Can you work these out from the model? Positions are in its coordinate system, mm. A direction names the side the tool comes from. Round coordinates to 2 decimals unless told otherwise and drop trailing zeros. Order: outer loops, then holes, each group sorted by start corner. A loop starts at its lowest first (then second) coordinate and runs counter-clockwise, first axis right, second up. Notation, with made-up numbers: M -16.75,42.5 L 29.25,42.5 A22 ccw 29.25,64.5 Z; hole C -17.75,4 d7. An arc over 180 degrees is marked long. One line per question, with ' | ' between items.
```python
from build123d import *

# Parameters (mm, degrees)
SKIZZE1_R                        = 2.5
AUFSATZ_LINEAR_AUSTRAGEN4_DEPTH  = 1
SKIZZE1_3_R                      = 2.5
SKIZZE1_3_R_2                    = 1.5
AUFSATZ_LINEAR_AUSTRAGEN5_DEPTH  = 10
SKIZZE1_4_R                      = 1.5
AUFSATZ_LINEAR_AUSTRAGEN6_DEPTH  = 12
VERRUNDUNG4_R                    = 1
SKIZZE1_5_W                      = 2
SKIZZE1_5_H                      = 16
AUFSATZ_LINEAR_AUSTRAGEN7_DEPTH  = 12
FASE3_SIZE                       = 12
VERRUNDUNG5_R                    = 12
SCHNITT_LINEAR_AUSTRAGEN2_DEPTH  = 12
SKIZZE5_4_R                      = 4.25
SKIZZE5_4_R_2                    = 3.45
AUFSATZ_LINEAR_AUSTRAGEN10_DEPTH = 6


with BuildPart() as part:
    # Skizze1 → Aufsatz-Linear austragen4 (new body)
    with BuildSketch(Plane.XY):
        with BuildLine():
            Line((-11, 12), (-16.5, 12))
            Line((-16.5, 12), (-16.5, 8))
            ThreePointArc((-16.5, 8), (-14.5, 6), (-16.5, 4))
            Line((-16.5, 4), (-16.5, -30))
            Line((-16.5, -30), (16.5, -30))
            Line((16.5, -30), (16.5, 4))
            ThreePointArc((16.5, 4), (14.5, 6), (16.5, 8))
            Line((16.5, 8), (16.5, 12))
            Line((16.5, 12), (11, 12))
            Line((11, 12), (9, 12))
            Line((9, 12), (9, 28))
            Line((9, 28), (-9, 28))
            Line((-9, 28), (-9, 12))
            Line((-9, 12), (-11, 12))
        make_face()
        with Locations((-11.5, -14)):
            Circle(SKIZZE1_R, mode=Mode.SUBTRACT)
        with Locations((11.5, -14)):
            Circle(SKIZZE1_R, mode=Mode.SUBTRACT)
        with Locations((-11.5, 9)):
            Circle(SKIZZE1_R, mode=Mode.SUBTRACT)
        with Locations((11.5, 9)):
            Circle(SKIZZE1_R, mode=Mode.SUBTRACT)
    extrude(amount=AUFSATZ_LINEAR_AUSTRAGEN4_DEPTH)

    # Skizze1<3> → Aufsatz-Linear austragen5 (add)
    # profile 1 of 4: a face of its own
    with BuildSketch(Plane.XY):
        with Locations((11.5, 9)):
            Circle(SKIZZE1_3_R)
        with Locations((11.5, 9)):
            Circle(SKIZZE1_3_R_2, mode=Mode.SUBTRACT)
    # profile 2 of 4: a face of its own
    with BuildSketch(Plane.XY):
        with Locations((-11.5, 9)):
            Circle(SKIZZE1_3_R)
        with Locations((-11.5, 9)):
            Circle(SKIZZE1_3_R_2, mode=Mode.SUBTRACT)
    # profile 3 of 4: a face of its own
    with BuildSketch(Plane.XY):
        with Locations((-11.5, -14)):
            Circle(SKIZZE1_3_R)
        with Locations((-11.5, -14)):
            Circle(SKIZZE1_3_R_2, mode=Mode.SUBTRACT)
    # profile 4 of 4: a face of its own
    with BuildSketch(Plane.XY):
        with Locations((11.5, -14)):
            Circle(SKIZZE1_3_R)
        with Locations((11.5, -14)):
            Circle(SKIZZE1_3_R_2, mode=Mode.SUBTRACT)
    extrude(amount=AUFSATZ_LINEAR_AUSTRAGEN5_DEPTH)

    # Skizze1<4> → Aufsatz-Linear austragen6 (add)
    with BuildSketch(Plane.XY):
        with Locations((-11.5, 9)):
            Circle(SKIZZE1_4_R)
        with Locations((11.5, 9)):
            Circle(SKIZZE1_4_R)
        with Locations((-11.5, -14)):
            Circle(SKIZZE1_4_R)
        with Locations((11.5, -14)):
            Circle(SKIZZE1_4_R)
    extrude(amount=AUFSATZ_LINEAR_AUSTRAGEN6_DEPTH)

    # Verrundung4
    verrundung4_edges = [part.edges().sort_by_distance(p)[0] for p in [
        (-13, 9, 12),
        (10, 9, 12),
        (-13, -14, 12),
        (10, -14, 12),
    ]]
    fillet(verrundung4_edges, radius=VERRUNDUNG4_R)

    # Skizze1<5> → Aufsatz-Linear austragen7 (add)
    with BuildSketch(Plane.XY):
        with Locations((-10, 20)):
            Rectangle(SKIZZE1_5_W, SKIZZE1_5_H)
        Polygon((11, 30), (-11, 30), (-11, 28), (-9, 28), (9, 28), (11, 28), align=None)
        with Locations((10, 20)):
            Rectangle(SKIZZE1_5_W, SKIZZE1_5_H)
    extrude(amount=AUFSATZ_LINEAR_AUSTRAGEN7_DEPTH)

    # Fase3
    # the kernel refuses this chamfer: 12 mm, written as the material it takes off along each edge
    with BuildSketch(Plane(origin=(-41.860195856, 12, 12), x_dir=(0, -0.027495876610586348, -0.9996219169112968), z_dir=(1, 0, 0))) as fase3_piece_1_section:
        Polygon((FASE3_SIZE * 0.999621916911, FASE3_SIZE * 0.0274958766106), (-FASE3_SIZE * 0.0274958766106, FASE3_SIZE * 0.999621916911), (0, 0), align=None)
    fase3_piece_1 = extrude(amount=63.720391711, mode=Mode.PRIVATE)
    fase3_piece_1 = split(fase3_piece_1, bisect_by=Plane(origin=(-10, 16.015873454, 1), z_dir=(0, 0, 1)), keep=Keep.TOP, mode=Mode.PRIVATE)
    add(fase3_piece_1, mode=Mode.SUBTRACT)
    with BuildSketch(Plane(origin=(-21.860195856, 12, 12), x_dir=(0, -0.027495876610586348, -0.9996219169112968), z_dir=(1, 0, 0))) as fase3_piece_2_section:
        Polygon((FASE3_SIZE * 0.999621916911, FASE3_SIZE * 0.0274958766106), (-FASE3_SIZE * 0.0274958766106, FASE3_SIZE * 0.999621916911), (0, 0), align=None)
    fase3_piece_2 = extrude(amount=63.720391711, mode=Mode.PRIVATE)
    fase3_piece_2 = split(fase3_piece_2, bisect_by=Plane(origin=(10, 16.015873454, 1), z_dir=(0, 0, 1)), keep=Keep.TOP, mode=Mode.PRIVATE)
    add(fase3_piece_2, mode=Mode.SUBTRACT)

    # Verrundung5
    verrundung5_edges = [part.edges().sort_by_distance(p)[0] for p in [
        (-10, 24, 12),
    ]]
    fillet(verrundung5_edges, radius=VERRUNDUNG5_R)

    # Skizze5 → Schnitt-Linear austragen2 (cut)
    with BuildSketch(Plane(origin=(0, 30, 0), x_dir=(1, 0, 0), z_dir=(0, 1, 0))):
        with BuildLine():
            ThreePointArc((3.45, -6), (2.439518395, -3.560481605), (0, -2.55))
            Line((0, -2.55), (0, -9.45))
            ThreePointArc((0, -9.45), (2.439518395, -8.439518395), (3.45, -6))
        make_face()
        with BuildLine():
            Line((0, -9.45), (0, -2.55))
            ThreePointArc((0, -2.55), (-3.45, -6), (0, -9.45))
        make_face()
    extrude(amount=-SCHNITT_LINEAR_AUSTRAGEN2_DEPTH, mode=Mode.SUBTRACT)

    # Skizze5<4> → Aufsatz-Linear austragen10 (add)
    with BuildSketch(Plane(origin=(0, 30, 0), x_dir=(1, 0, 0), z_dir=(0, 1, 0))):
        with Locations(Location((0, -6, 0), (0, 0, 270))):
            Circle(SKIZZE5_4_R)
        with Locations(Location((0, -6, 0), (0, 0, 270))):
            Circle(SKIZZE5_4_R_2, mode=Mode.SUBTRACT)
    extrude(amount=-AUFSATZ_LINEAR_AUSTRAGEN10_DEPTH)


solid = part.part
```
(1) If we section it at C-C on y = 14.5: Please give me the cut outline in (x, z).
Final values:
outline: M -11,0 L 11,0 L 11,2.5 L 9,2.5 L 9,1 L -9,1 L -9,2.5 L -11,2.5 Z
(2) Will these pins go through, and if not, where does the flat tip stop? pin 1 Ø6 at (y, z) = (17, 6.5) entering from -X; pin 2 Ø6 at (y, z) = (6, 4.5) entering from -X; pin 3 Ø0.8 at (x, z) = (-13.5, 0.5) entering from +Y.
Final values:
pin 1: x = -11 | pin 2: x = -14 | pin 3: y = 12
(3) Thinking about a two-plate mould opening in Y: for faces 4 (the flat face through (-11, 23, 5)), 5 (the flat face through (13, 8, 10)), 6 (the flat face through (-2, 28, 10)), which applies, released by +Y, released by -Y, zero draft, split by the parting line, or undercut?
Final values:
face 4: zero draft | face 5: undercut | face 6: released by -Y
(4) If we section it at A-A on z = 6: Please give me the cut outline in (x, y), plus the area to 3 significant figures.
Final values:
outline: C -11.5,-14 d5; C -11.5,9 d5; M -11,18 L -9,18 L -9,28 L -4.25,28 L -4.25,24 L -3.45,24 L -3.45,30 L -11,30 Z; M 3.45,24 L 4.25,24 L 4.25,28 L 9,28 L 9,18 L 11,18 L 11,30 L 3.45,30 Z; C 11.5,-14 d5; C 11.5,9 d5 | area: 155 mm^2
(5) If we section it at D-D on x = -6: Please give me the cut outline in (y, z), plus the area to 3 significant figures.
Final values:
outline: M -30,0 L 30,0 L 30,12 L 28.97,12 A12 ccw 28,11.96 L 28,1 L -30,1 Z | area: 82.0 mm^2
(6) If we section it at B-B on x = 0: Please give me the cut outline in (y, z).
Final values:
outline: M -30,0 L 30,0 L 30,2.55 L 24,2.55 L 24,1.75 L 28,1.75 L 28,1 L -30,1 Z; M 24,9.45 L 30,9.45 L 30,12 L 28.97,12 A12 ccw 28,11.96 L 28,10.25 L 24,10.25 Z
(7) Please list where these lines run through material, in increasing order: probe 1 along X at (y, z) = (25.95, 6); probe 2 along Y at (x, z) = (13.5, 8.5); probe 3 along Z at (x, y) = (12, -16). Write a range as [from, to].
Final values:
probe 1: [-11, -9], [-4.25, -3.45], [3.45, 4.25], [9, 11] | probe 2: [-15.5, -12.5], [7.5, 10.5] | probe 3: [0, 10]
(8) On a 3-axis mill with a long thin cutter (end or side, diameter ignored), from which of +Z, -Z, +X, -X, +Y, -Y can I reach the whole of each face in a straight line? I mean faces 1 (the flat face through (0, 0, 0)), 2 (the flat face through (3, 24, 4)), 3 (the flat face through (13, -15, 10)). Say none if no direction works.
Final values:
face 1: -Z, +X, -X, +Y, -Y | face 2: +Z, -Y | face 3: +Z
